Study the drawing (mm; zero at the part's minimum x, y, z) and answer. A direction names the side the tool comes from. Coordinates: 2 decimals unless noted, no trailing zeros. Loops run counter-clockwise (first coordinate to the right, second up) from the corner with the lowest first, then second, coordinate; pieces in that order, holes last. Notation, with made-up numbers: (45, 86) -> (87, 86) arc R31 ccw to (87, 118) -> close; hole circle Ø10 at (28.5, 4). An arc over 180 degrees is marked (long way). Answer as a JSON object with one key per item and string values. Group by question number.
Q1. Each of these flat-tipped pins is pushed along its axis until it touches: P1, Ø5, axis at x = 39.27, y = 12.38, coming from the -Z side; P2, Ø5, axis at x = 27.5, z = 2, coming from the -Y side; P3, Ø2, axis at y = 37, z = 11.5, coming from the +X side (1 decimal). Where does it stop, or does it pass through?
Q2. For the marked faces 1 and 2, determine the directions among +Z, -Z, +X, -X, +Y, -Y from which every point of the face is accessible in a straight line to the end or side of a thin tool.
Q3. The part is cut by section B-B on y = 41.5. Write down the section's boundary in (x, z), and give its area (3 significant figures).
Q4. Determine the mould class of the marked faces 3, 4 and 5 for opening direction Y: released by +Y, released by -Y, zero draft, split by the parting line, or undercut.
Q5. Straight lines are drawn through the part: line 1 along X through (y, z) = (12.5, 9) (1 decimal); line 2 along Z through (x, y) = (7, 33.5); line 3 along X through (y, z) = (41.91, 10.75) (1 decimal). For each, find the intervals that lie inside material, in ascending order. Write a range as [from, to].
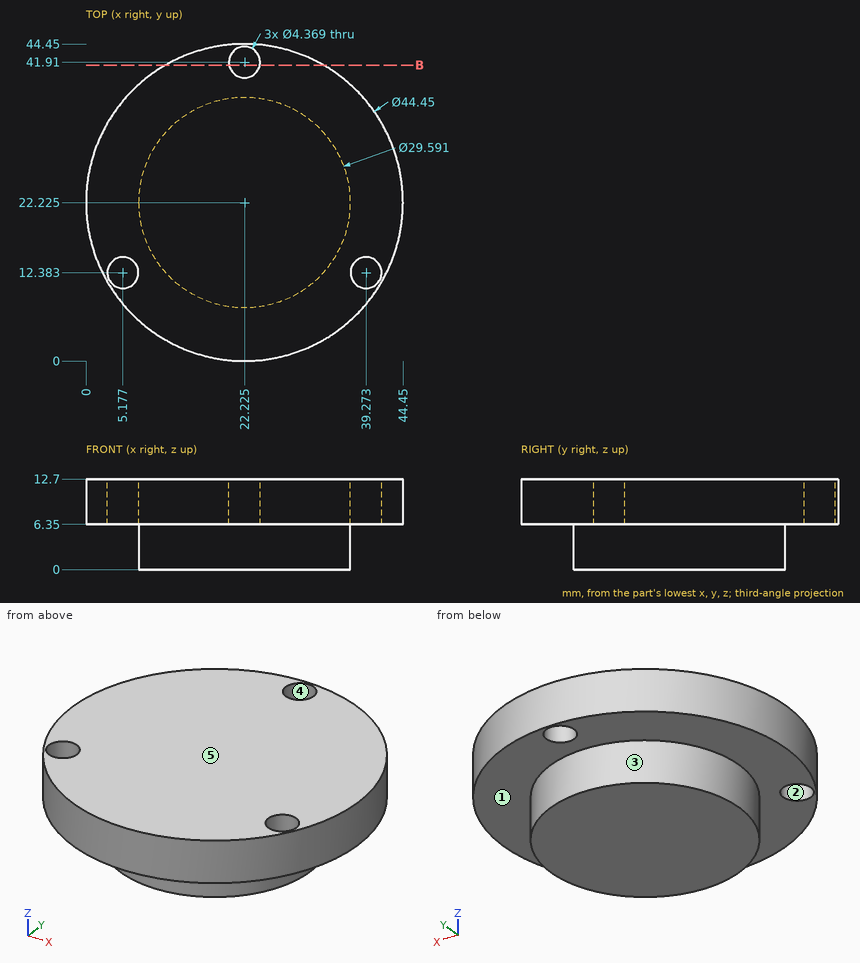
Final values:
{
 "1": {"P1": "stops at z = 6.35", "P2": "stops at y = 7.69", "P3": "stops at x = 39.7"},
 "2": {"face 1": "-Z", "face 2": "+Z, -Z"},
 "3": {"outline": "(11.16, 6.35) -> (20.08, 6.35) -> (20.08, 12.7) -> (11.16, 12.7) -> close; (24.37, 6.35) -> (33.29, 6.35) -> (33.29, 12.7) -> (24.37, 12.7) -> close", "area": "113 mm2"},
 "4": {"face 3": "split by the parting line", "face 4": "undercut", "face 5": "zero draft"},
 "5": {"line 1": "x = [2.2, 3], [7.4, 37.1], [41.5, 42.2]", "line 2": "z = [6.35, 12.7]", "line 3": "x = [11.9, 20], [24.4, 32.5]"}
}
